from build123d import *

# Parameters (mm, degrees)
STOCK_BATTERY_BASE_1_DEPTH   = 7.5
STOCK_BATTERY_BASE_1_2_DEPTH = 4.5
BOSS_EXTRUDE1_DEPTH          = 2.5
BOSS_EXTRUDE2_DEPTH          = 7
SKETCH3_R                    = 2.5
BOSS_EXTRUDE4_DEPTH          = 3
SKETCH4_R                    = 1.25
BOSS_EXTRUDE5_DEPTH          = 3


# Read off the part's stored shape, not the designer's step: Stock-battery base-1
with BuildPart() as part:
    # Stock-battery base-1 outline → Stock-battery base-1 (new body)
    with BuildSketch(Plane.XY):
        with BuildLine():
            Line((16.459100066, -58.832087736), (16.459100066, 43.22938712))
            Line((16.459100066, 43.22938712), (0.459100066, 44.038083245))
            Line((0.459100066, 44.038083245), (0.459100066, 47.61329436))
            Line((0.459100066, 47.61329436), (-75.963345356, 51.475952827))
            add(Edge.make_bspline(
                [(-75.963345356, 51.475952827), (-76.969760945, 51.385311169), (-77.956664013, 51.213742336), (-79.395866789, 50.78571401), (-79.86970863, 50.613871194), (-80.796837185, 50.204577199), (-81.240590365, 49.971323111), (-82.089787414, 49.449496549), (-82.495246976, 49.160946736), (-83.271465049, 48.533739024), (-83.643007435, 48.194375714), (-84.708444042, 47.116795042), (-85.333215001, 46.343374139), (-86.491296884, 44.737676097), (-87.023827607, 43.904896882), (-88.044872363, 42.211012893), (-88.533034054, 41.34968138), (-89.982900727, 38.756279626), (-90.93240726, 37.013628654), (-92.999467157, 33.650383947), (-94.114586107, 32.031232641), (-95.60337212, 30.287705281), (-95.819744565, 30.042891916), (-96.040899934, 29.801740739)],
                knots=[0, 0, 0, 0, 0.0625, 0.0625, 0.09375, 0.09375, 0.125, 0.125, 0.15625, 0.15625, 0.1875, 0.1875, 0.25, 0.25, 0.3125, 0.3125, 0.375, 0.375, 0.5, 0.5, 0.625, 0.625, 0.645748558, 0.645748558, 0.645748558, 0.645748558], degree=3))
            Line((-96.040899934, 29.801740739), (-101.040899934, 29.801740739))
            Line((-101.040899934, 29.801740739), (-101.040899934, -41.829259963))
            Line((-101.040899934, -41.829259963), (-96.040899934, -41.829259963))
            add(Edge.make_bspline(
                [(-96.040899934, -41.829259963), (-95.798899268, -42.093160096), (-95.56197213, -42.362136183), (-94.03954966, -44.156758027), (-92.923608678, -45.792412437), (-90.858487716, -49.170948695), (-89.911065512, -50.914960796), (-88.457766632, -53.51029646), (-87.967520262, -54.371999904), (-86.940892781, -56.06392928), (-86.404912323, -56.894254814), (-85.530671439, -58.091259413), (-85.227414802, -58.482089731), (-84.588818098, -59.241614046), (-84.254184704, -59.609132259), (-83.204929916, -60.651600397), (-82.440569541, -61.270576891), (-81.160629249, -62.042718444), (-80.719255742, -62.269433113), (-79.817314106, -62.660888928), (-79.3554021, -62.826549047), (-77.940467092, -63.243286827), (-76.954208328, -63.414201398), (-75.963345356, -63.503442328)],
                knots=[0.352672192, 0.352672192, 0.352672192, 0.352672192, 0.375, 0.375, 0.5, 0.5, 0.625, 0.625, 0.6875, 0.6875, 0.75, 0.75, 0.78125, 0.78125, 0.8125, 0.8125, 0.875, 0.875, 0.90625, 0.90625, 0.9375, 0.9375, 1, 1, 1, 1], degree=3))
            Line((-75.963345356, -63.503442328), (16.459100066, -58.832087736))
        make_face()
    extrude(amount=STOCK_BATTERY_BASE_1_DEPTH)

    # Stock-battery base-1 2 outline → Stock-battery base-1 2 (add)
    with BuildSketch(Plane.XY):
        Polygon((16.459100066, 43.22938712), (16.459100066, 46.804598235), (0.459100066, 47.61329436), (0.459100066, 44.038083245), align=None)
    extrude(amount=STOCK_BATTERY_BASE_1_2_DEPTH)

    # Sketch1 → Boss-Extrude1 (add)
    with BuildSketch(Plane(origin=(16.459100066, 0, 0), x_dir=(0, 0, -1), z_dir=(1, 0, 0))):
        Polygon((0, -58.832087736), (0, 46.804598235), (-4.5, 46.804598235), (-4.5, 43.22938712), (-7.5, 43.22938712), (-7.5, -58.832087736), align=None)
    extrude(amount=BOSS_EXTRUDE1_DEPTH)

    # Sketch2 → Boss-Extrude2 (add)
    with BuildSketch(Plane(origin=(18.959100066, 0, 0), x_dir=(0, 0, -1), z_dir=(1, 0, 0))):
        Polygon((-2.3, 41.02938712), (-2.2, 41.02938712), (-2.2, -56.632087736), (-5.3, -56.632087736), (-5.3, 41.02938712), align=None)
    extrude(amount=BOSS_EXTRUDE2_DEPTH)

    # Sketch3 → Boss-Extrude4 (add)
    with BuildSketch(Plane.XY.offset(7.5)):
        with Locations(Location((-72.963345356, 36.964917072, 0), (0, 0, 180))):
            Circle(SKETCH3_R)
        with Locations(Location((-14.960454045, 36.964917072, 0), (0, 0, 180))):
            Circle(SKETCH3_R)
        with Locations(Location((-14.960454045, -48.992436296, 0), (0, 0, 180))):
            Circle(SKETCH3_R)
        with Locations(Location((-72.963345356, -48.992436296, 0), (0, 0, 180))):
            Circle(SKETCH3_R)
    extrude(amount=BOSS_EXTRUDE4_DEPTH)

    # Sketch4 → Boss-Extrude5 (add)
    with BuildSketch(Plane.XY.offset(10.5)):
        with Locations((-72.963345356, 36.964917072)):
            Circle(SKETCH4_R)
        with Locations((-14.960454045, 36.964917072)):
            Circle(SKETCH4_R)
        with Locations((-72.963345356, -48.992436296)):
            Circle(SKETCH4_R)
        with Locations((-14.960454045, -48.992436296)):
            Circle(SKETCH4_R)
    extrude(amount=BOSS_EXTRUDE5_DEPTH)


solid = part.part
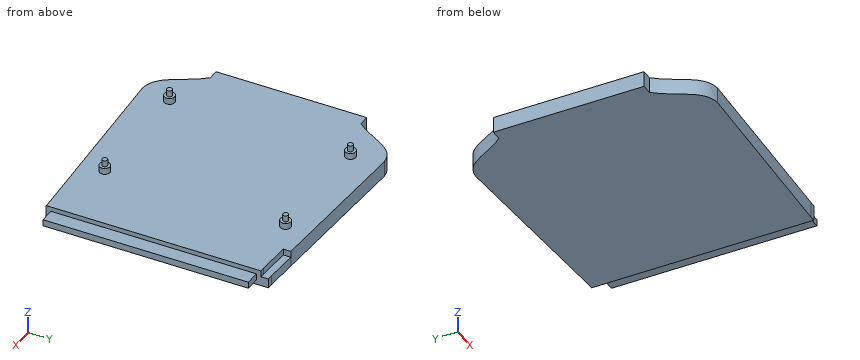
Geometry: final body of the model. Coordinates: model frame, mm. Coordinates: 2 decimals unless noted, no trailing zeros. Order: outer loops, then holes, each group sorted by start corner. A loop starts at its lowest first (then second) coordinate and runs counter-clockwise, first axis right, second up. Notation, with made-up numbers: M 30,37.5 L 34,37.5 A22 cw 34,43.5 Z; hole C 71.5,52 d6. An arc over 180 degrees is marked long. One line per question, with ' | ' between items. Start each with the question number.
Item 1: Cut plane B-B, the plane x = -9. Return the cut outline in (y, z).
Item 2: Pin query (flat end, axial travel): pin 1 Ø1.5 at (y, z) = (-48.5, 2.5) entering from -X; pin 2 Ø0.9 at (x, z) = (22.5, 3) entering from -Y; pin 3 Ø3 at (x, z) = (18, 2) entering from +Y. Return the tip coordinate at first contact, or that it passes through.
Item 3: Ray query, probe 1 along Y at (x, z) = (-73, 11.5); probe 2 along Z at (x, y) = (-8.5, -41); probe 3 along X at (y, z) = (24, 2). Return the intervals inside material, ascending. Write a range as [from, to].
Item 4: Cut plane C-C, the plane x = -58.5. Return the cut outline in (y, z), then the cut area to 3 significant figures.
Item 5: Cut plane A-A, the plane y = -16. Return the cut outline in (x, z), then the cut area to 3 significant figures.
A:
1) outline: M -60.12,0 L 48.09,0 L 48.09,7.5 L -60.12,7.5 Z
2) pin 1: stops at x = -91.73 | pin 2: stops at y = -56.63 | pin 3: stops at y = 46.8
3) probe 1: y = [-50.24, -47.74], [35.72, 38.21] | probe 2: z = [0, 7.5] | probe 3: x = [-101.04, 18.96]
4) outline: M -62.62,0 L 50.59,0 L 50.59,7.5 L -62.62,7.5 Z | area: 849 mm2
5) outline: M -101.04,0 L 18.96,0 L 18.96,2.2 L 25.96,2.2 L 25.96,5.3 L 18.96,5.3 L 18.96,7.5 L -101.04,7.5 Z | area: 922 mm2
